```python
from build123d import *

# Parameters (mm, degrees)
SKETCH1_W                    = 346.075
SKETCH1_H                    = 482.6
BOSS_EXTRUDE1_DEPTH          = 6.35
FILLET1_R                    = 6.35
F_3_8_0_375_DIAMETER_HOLE1_D = 9.525


with BuildPart() as part:
    # Sketch1 → Boss-Extrude1 (new body)
    with BuildSketch(Plane(origin=(0, 0, 0), x_dir=(1, 0, 0), z_dir=(0, 1, 0))):
        Rectangle(SKETCH1_W, SKETCH1_H)
    extrude(amount=BOSS_EXTRUDE1_DEPTH)

    # Fillet1
    fillet1_edges = [part.edges().sort_by_distance(p)[0] for p in [
        (173.0375, 3.175, 241.3),
        (-173.0375, 3.175, 241.3),
        (-173.0375, 3.175, -241.3),
        (173.0375, 3.175, -241.3),
    ]]
    fillet(fillet1_edges, radius=FILLET1_R)

    # 3/8 (0.375) Diameter Hole1 (through all)
    with Locations(Plane(origin=(0, 6.35, 0), x_dir=(1, 0, 0), z_dir=(0, 1, 0))):
        with Locations((-127, 209.55), (127, 209.55)):
            Hole(F_3_8_0_375_DIAMETER_HOLE1_D / 2)


solid = part.part
```
Source: CAD feature listing. Evaluate the final solid. Frame: model axes, mm. Coordinates: 2 decimals unless noted, no trailing zeros. Loops run counter-clockwise (first coordinate to the right, second up) from the corner with the lowest first, then second, coordinate; pieces in that order, holes last. Notation, with made-up numbers: M 3.25,-9.75 L 55.25,-9.75 A14 cw 55.25,5.25 Z; hole C 13,-14 d2. An arc over 180 degrees is marked long. Use a Markdown table: item, result. Add a question column.
Q1. Section query A-A, the plane z = -209.55. Return loops of the section in (x, y).
Q2. Draft query along X for faces 1 (the cylindrical face through (127.62, 3.13, -214.27)), 2 (the flat face through (-2, 6.35, -3)), 3 (the cylindrical face through (-126.38, 3.13, -214.27)). Return one class per face: pulls with the +X half, pulls with the -X half, needs draft (parallel to the pull), parting line crosses it, or undercut.
Q3. First-contact query: pin 1 (5.5 mm diameter, centred on x = 127, z = -209.55, fed in from +Y). Flat tip, straight axial feed; report the tip coordinate or a pass-through.
Q4. Section query B-B, the plane x = 127. Return loops of the section in (y, z), and give its area (3 significant figures).
Q5. Material intervals for L1, parallel to X at y = 2.25, z = -209.55; L2, parallel to Z at x = 127, y = 4.5; L3, parallel to Z at x = -124, y = 4.75, sorted ascending.
Result:
| question | item | result |
|---|---|---|
| 1 | outline | M -173.04,0 L -131.76,0 L -131.76,6.35 L -173.04,6.35 Z; M -122.24,0 L 122.24,0 L 122.24,6.35 L -122.24,6.35 Z; M 131.76,0 L 173.04,0 L 173.04,6.35 L 131.76,6.35 Z |
| 2 | face 1 | undercut |
| 2 | face 2 | needs draft |
| 2 | face 3 | undercut |
| 3 | pin 1 | passes through |
| 4 | outline | M 0,-241.3 L 6.35,-241.3 L 6.35,-214.31 L 0,-214.31 Z; M 0,-204.79 L 6.35,-204.79 L 6.35,241.3 L 0,241.3 Z |
| 4 | area | 3,000 mm2 |
| 5 | L1 | x = -173.04 to -131.76, -122.24 to 122.24, 131.76 to 173.04 |
| 5 | L2 | z = -241.3 to -214.31, -204.79 to 241.3 |
| 5 | L3 | z = -241.3 to -213.25, -205.85 to 241.3 |
